from build123d import *

# Parameters (mm, degrees)
BRACKET_FOOT_PROFILE_W                    = 16
BRACKET_FOOT_PROFILE_H                    = 11.75
BRACKET_FOOT_DEPTH                        = 4
UPRIGHT_START                             = 4
UPRIGHT_PROFILE_W                         = 16
UPRIGHT_PROFILE_H                         = 5.75
UPRIGHT_DEPTH                             = 46.45
UPPER_START                               = 46.65
UPPER_ARM_PROFILE_W                       = 16
UPPER_ARM_PROFILE_H                       = 13.2
UPPER_ARM_DEPTH                           = 3.8
BRACKET_START                             = -0.1
BRACKET_BOLT_CLEARANCES_PROFILE_R         = 1.65
BRACKET_BOLT_CLEARANCES_DEPTH             = 4.2
INTEGRAL_START                            = 43.35
INTEGRAL_STOP_PIN_DIAMETER_4_MM_PROFILE_R = 2
INTEGRAL_STOP_PIN_DIAMETER_4_MM_DEPTH     = 3.5


with BuildPart() as part:
    # Bracket foot profile → Bracket foot (new body)
    with BuildSketch(Plane.XY):
        with Locations((0, 33.125)):
            Rectangle(BRACKET_FOOT_PROFILE_W, BRACKET_FOOT_PROFILE_H)
    extrude(amount=BRACKET_FOOT_DEPTH)

    # Upright profile → Upright (add)
    with BuildSketch(Plane.XY.offset(UPRIGHT_START)):
        with Locations((0, 30.125)):
            Rectangle(UPRIGHT_PROFILE_W, UPRIGHT_PROFILE_H)
    extrude(amount=UPRIGHT_DEPTH)

    # Upper arm profile → Upper arm (add)
    with BuildSketch(Plane.XY.offset(UPPER_START)):
        with Locations((0, 21.1)):
            Rectangle(UPPER_ARM_PROFILE_W, UPPER_ARM_PROFILE_H)
    extrude(amount=UPPER_ARM_DEPTH)

    # Bracket bolt clearances profile → Bracket bolt clearances (cut)
    with BuildSketch(Plane.XY.offset(BRACKET_START)):
        with Locations((-4.5, 36)):
            Circle(BRACKET_BOLT_CLEARANCES_PROFILE_R)
        with Locations((4.5, 36)):
            Circle(BRACKET_BOLT_CLEARANCES_PROFILE_R)
    extrude(amount=BRACKET_BOLT_CLEARANCES_DEPTH, mode=Mode.SUBTRACT)

    # Integral stop pin diameter 4 mm profile → Integral stop pin diameter 4 mm (add)
    with BuildSketch(Plane.XY.offset(INTEGRAL_START)):
        with Locations((0, 17)):
            Circle(INTEGRAL_STOP_PIN_DIAMETER_4_MM_PROFILE_R)
    extrude(amount=INTEGRAL_STOP_PIN_DIAMETER_4_MM_DEPTH)


solid = part.part
Design review of the part built by this model. Coordinates are the model's own, in mm. A direction names the side the tool comes from. Coordinates: 2 decimals unless noted, no trailing zeros. Order: outer loops, then holes, each group sorted by start corner. A loop starts at its lowest first (then second) coordinate and runs counter-clockwise, first axis right, second up.
Item 1: Take a section at C-C, the plane z = 3. Write out the cut boundary in (x, y).
Item 2: For pin 1 Ø5 at (x, z) = (-4.5, 18) entering from +Y; pin 2 Ø3 at (x, y) = (1, 36) entering from +Z; pin 3 Ø4.5 at (x, y) = (1, 17.5) entering from -Z, all flat-tipped, find the tip position at first contact; note any pin that passes through.
Item 3: For line 1 (X direction, y = 36, z = 3); line 2 (Y direction, x = -4.5, z = 3.1); line 3 (Y direction, x = -5.25, z = 33), list the stretches that pass through material, from the lowest coordinate up.
Item 4: Take a section at D-D, the plane y = 17. Write out the cut boundary in (x, z).
Item 5: The part is to be moulded in two halves that separate along X. For faces 1 (the flat face through (0, 24, 50.45)), 2 (the flat face through (-8, 29, 29)), 3 (the cylindrical face through (-5.716, 37.115, 1.972)), say which applies: pulls with the +X half, pulls with the -X half, needs draft (parallel to the pull), parting line crosses it, or undercut.
Item 6: Take a section at A-A, the plane x = 4.5. Write out the cut boundary in (y, z).
Item 7: Take a section at B-B, the plane y = 36. Write out the cut boundary in (x, z).
Item 8: For faces 4 (the cylindrical face through (0, 19, 45)), 5 (the flat face through (0, 17, 43.35)), 6 (the flat face through (0, 33, 27)), list the 3-axis set-ups (+Z, -Z, +X, -X, +Y, -Y) from which the entire face can be reached by the end or side of a thin tool; tool diameter is ignored.
The answers:
1. outline: (-8, 27.25) - (8, 27.25) - (8, 39) - (-8, 39) - close; hole circle Ø3.3 at (-4.5, 36); hole circle Ø3.3 at (4.5, 36)
2. pin 1: stops at y = 33
2. pin 2: stops at z = 4
2. pin 3: stops at z = 43.35
3. line 1: x = -8 to -6.15, -2.85 to 2.85, 6.15 to 8
3. line 2: y = 27.25 to 34.35, 37.65 to 39
3. line 3: y = 27.25 to 33
4. outline: (-8, 46.65) - (-2, 46.65) - (-2, 43.35) - (2, 43.35) - (2, 46.65) - (8, 46.65) - (8, 50.45) - (-8, 50.45) - close
5. face 1: needs draft
5. face 2: pulls with the -X half
5. face 3: undercut
6. outline: (14.5, 46.65) - (27.25, 46.65) - (27.25, 0) - (34.35, 0) - (34.35, 4) - (33, 4) - (33, 50.45) - (14.5, 50.45) - close; (37.65, 0) - (39, 0) - (39, 4) - (37.65, 4) - close
7. outline: (-8, 0) - (-6.15, 0) - (-6.15, 4) - (-8, 4) - close; (-2.85, 0) - (2.85, 0) - (2.85, 4) - (-2.85, 4) - close; (6.15, 0) - (8, 0) - (8, 4) - (6.15, 4) - close
8. face 4: -Z
8. face 5: -Z, +X, -X, -Y
8. face 6: +Z, +X, -X, +Y
